Can you work these out from the model? Positions are in its coordinate system, mm. Face numbers are marked on the shaded views. A direction names the side the tool comes from. Round coordinates to 2 decimals unless told otherwise and drop trailing zeros. Write each loop counter-clockwise with the first axis right and the second up, starting at its lowest first coordinate (ties: lowest second). Pieces come first, ordered by that corner, then holes. Notation, with made-up numbers: M 10,13 L 46,13 A12 ccw 46,20 Z; hole C -19,33.5 d8. An arc over 180 degrees is marked long. Answer as a JSON object with one key per item and string values. Group by question number.
1) Suppose I cut it at D-D, the plane z = 17. Write out the boundary of the cut face in (x, y), and give its area (3 significant figures).
2) Suppose I cut it at A-A, the plane y = 0. Write out the boundary of the cut face in (x, z), and give its area (3 significant figures).
3) Suppose I cut it at C-C, the plane x = -17. Write out the boundary of the cut face in (y, z).
4) If we mould it in two halves opening along X, with no side actions, what happens to the marked faces 1, 2 and 3? For each: +X half, -X half, draft (parallel to the pull), parting line (faces both ways), or undercut.
5) On a 3-axis mill with a long thin cutter (end or side, diameter ignored), from which of +Z, -Z, +X, -X, +Y, -Y can I reach the whole of each face in a straight line? I mean the marked faces 4 and 5. Say none if no direction works.
6) I'm going to push flat-ended pins straight in: pin 1 Ø2 at (x, y) = (-4.5, -3.5) entering from +Z; pin 2 Ø8 at (x, y) = (-16.5, -10) entering from -Z; pin 3 Ø9 at (y, z) = (0, -20.05) entering from +X; pin 4 Ø1 at (x, y) = (-10.5, -4) entering from -Z. Where does each tip first touch, or does it pass through?
7) Please list where these lines run through material, in increasing order: L1, parallel to Y at x = -10, z = 11.5; L2, parallel to Z at x = -15.25, y = 5.5; L3, parallel to Y at x = -8, z = -5.5. Write a range as [from, to].
8) Suppose I cut it at B-B, the plane z = 10. Write out the boundary of the cut face in (x, y).
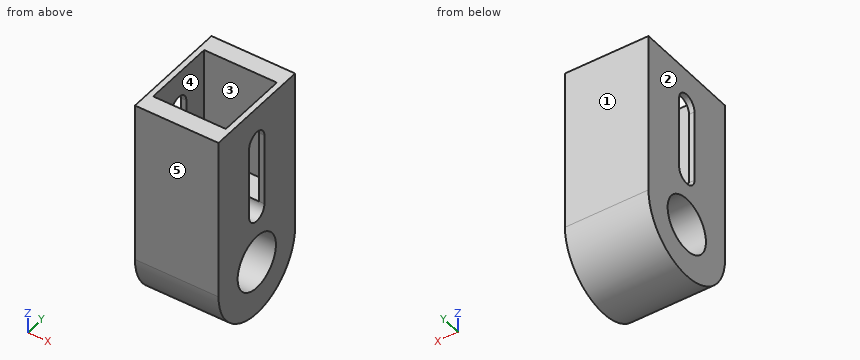
from build123d import *

# Parameters (mm, degrees)
BOSS_EXTRUDE1_DEPTH = 23
CUT_EXTRUDE1_DEPTH  = 45.52248299
SKETCH3_R           = 7.5
CUT_EXTRUDE2_DEPTH  = 45.52248299
SKETCH4_W           = 20
SKETCH4_H           = 20
CUT_EXTRUDE3_DEPTH  = 30


with BuildPart() as part:
    # Sketch1 → Boss-Extrude1 (new body)
    with BuildSketch(Plane(origin=(0, 0, 0), x_dir=(0, 0, -1), z_dir=(1, 0, 0))):
        with BuildLine():
            Line((-24.953580902, 15), (20.046419098, 15))
            ThreePointArc((20.046419098, 15), (35.046419098, 0), (20.046419098, -15))
            Line((20.046419098, -15), (-24.953580902, -15))
            Line((-24.953580902, -15), (-24.953580902, 15))
        make_face()
    extrude(amount=-BOSS_EXTRUDE1_DEPTH)

    # Sketch2 → Cut-Extrude1 (cut, through all)
    with BuildSketch(Plane(origin=(0, 0, 0), x_dir=(0, 0, -1), z_dir=(1, 0, 0))):
        with BuildLine():
            Line((-14.953580902, 3), (5.046419098, 3))
            ThreePointArc((5.046419098, 3), (8.046419098, 0), (5.046419098, -3))
            Line((5.046419098, -3), (-14.953580902, -3))
            ThreePointArc((-14.953580902, -3), (-17.953580902, 0), (-14.953580902, 3))
        make_face()
    extrude(amount=-CUT_EXTRUDE1_DEPTH, mode=Mode.SUBTRACT)

    # Sketch3 → Cut-Extrude2 (cut, through all)
    with BuildSketch(Plane(origin=(0, 0, 0), x_dir=(0, 0, -1), z_dir=(1, 0, 0))):
        with Locations((20.046419098, 0)):
            Circle(SKETCH3_R)
    extrude(amount=-CUT_EXTRUDE2_DEPTH, mode=Mode.SUBTRACT)

    # Sketch4 → Cut-Extrude3 (cut)
    with BuildSketch(Plane.XY.offset(24.953580902)):
        with Locations((-11.5, 0)):
            Rectangle(SKETCH4_W, SKETCH4_H)
    extrude(amount=-CUT_EXTRUDE3_DEPTH, mode=Mode.SUBTRACT)


solid = part.part
Results:
{
 "1": {"outline": "M -23,-15 L 0,-15 L 0,-2.19 L -1.5,-2.19 L -1.5,-10 L -21.5,-10 L -21.5,-2.19 L -23,-2.19 Z; M -23,2.19 L -21.5,2.19 L -21.5,10 L -1.5,10 L -1.5,2.19 L 0,2.19 L 0,15 L -23,15 Z", "area": "277 mm^2"},
 "2": {"outline": "M -23,-35.05 L 0,-35.05 L 0,-27.55 L -23,-27.55 Z; M -23,-12.55 L 0,-12.55 L 0,-8.05 L -23,-8.05 Z; M -23,17.95 L -21.5,17.95 L -21.5,24.95 L -23,24.95 Z; M -1.5,17.95 L 0,17.95 L 0,24.95 L -1.5,24.95 Z", "area": "297 mm^2"},
 "3": {"outline": "M -15,-20.05 A15 ccw 15,-20.05 L 15,24.95 L 10,24.95 L 10,-5.05 L 3,-5.05 A3 cw -3,-5.05 L -10,-5.05 L -10,24.95 L -15,24.95 Z; hole C 0,-20.05 d15"},
 "4": {"face 1": "draft", "face 2": "-X half", "face 3": "undercut"},
 "5": {"face 4": "+Z", "face 5": "+Z, -Z, +X, -X, -Y"},
 "6": {"pin 1": "z = -5.05", "pin 2": "z = -33.79", "pin 3": "through", "pin 4": "z = -34.63"},
 "7": {"L1": "[-15, -10], [10, 15]", "L2": "[-34, -25.15], [-14.95, -5.05]", "L3": "[-15, -2.97], [2.97, 15]"},
 "8": {"outline": "M -23,-15 L 0,-15 L 0,-3 L -1.5,-3 L -1.5,-10 L -21.5,-10 L -21.5,-3 L -23,-3 Z; M -23,3 L -21.5,3 L -21.5,10 L -1.5,10 L -1.5,3 L 0,3 L 0,15 L -23,15 Z"}
}
